from build123d import *

# Parameters (mm, degrees)
SKETCH1_W               = 300
SKETCH1_H               = 300
BOSS_EXTRUDE1_DEPTH     = 3
SKETCH2_W               = 300
SKETCH2_H               = 300
SKETCH2_W_2             = 294
SKETCH2_H_2             = 294
BOSS_EXTRUDE2_DEPTH     = 297
SKETCH3_W               = 300
SKETCH3_H               = 300
BOSS_EXTRUDE3_DEPTH     = 3
SKETCH4_R               = 25
CUT_EXTRUDE1_DEPTH      = 1
CUT_EXTRUDE1_DEPTH_BACK = 301
SKETCH5_W               = 300
SKETCH5_H               = 300
CUT_EXTRUDE2_DEPTH      = 3


with BuildPart() as part:
    # Sketch1 → Boss-Extrude1 (new body)
    with BuildSketch(Plane(origin=(0, 0, 0), x_dir=(1, 0, 0), z_dir=(0, 1, 0))):
        Rectangle(SKETCH1_W, SKETCH1_H)
    extrude(amount=BOSS_EXTRUDE1_DEPTH)

    # Sketch2 → Boss-Extrude2 (add)
    with BuildSketch(Plane(origin=(0, 3, 0), x_dir=(1, 0, 0), z_dir=(0, 1, 0))):
        Rectangle(SKETCH2_W, SKETCH2_H)
        Rectangle(SKETCH2_W_2, SKETCH2_H_2, mode=Mode.SUBTRACT)
    extrude(amount=BOSS_EXTRUDE2_DEPTH)

    # Sketch3 → Boss-Extrude3 (add)
    with BuildSketch(Plane(origin=(0, 300, 0), x_dir=(1, 0, 0), z_dir=(0, 1, 0))):
        Rectangle(SKETCH3_W, SKETCH3_H)
    extrude(amount=-BOSS_EXTRUDE3_DEPTH)

    # Sketch4 → Cut-Extrude1 (cut, two sides)
    with BuildSketch(Plane(origin=(150, 0, 0), x_dir=(0, 0, -1), z_dir=(1, 0, 0))) as cut_extrude1_sk:
        with Locations((0, 50)):
            Circle(SKETCH4_R)
    extrude(amount=CUT_EXTRUDE1_DEPTH, mode=Mode.SUBTRACT)
    extrude(cut_extrude1_sk.sketch, amount=-CUT_EXTRUDE1_DEPTH_BACK, mode=Mode.SUBTRACT)

    # Sketch5 → Cut-Extrude2 (cut)
    with BuildSketch(Plane.XZ):
        Rectangle(SKETCH5_W, SKETCH5_H)
    extrude(amount=-CUT_EXTRUDE2_DEPTH, mode=Mode.SUBTRACT)


solid = part.part
Design review of the part built by this model. Coordinates are the model's own, in mm. A direction names the side the tool comes from. Round coordinates to 2 decimals unless told otherwise and drop trailing zeros. Write each loop counter-clockwise with the first axis right and the second up, starting at its lowest first coordinate (ties: lowest second). Pieces come first, ordered by that corner, then holes. Notation, with made-up numbers: (85, 86) - (99, 86) arc R25 cw to (99, 113) - close; hole circle Ø5 at (-15.5, 79.25). An arc over 180 degrees is marked (long way). Return JSON: item names as keys, results as strings. Group by question number.
Item 1: We need section B-B on y = 50. Write out the cut boundary in (x, z), and give its area (3 significant figures).
Item 2: We need section D-D on y = 233. Write out the cut boundary in (x, z).
Item 3: The part is to be moulded in two halves that separate along Z. For faces 1 (the face through (-147, 148, 2)), 2 (the face through (-2, 149, 150)), 3 (the face through (-150, 149, 2)), say which applies: pulls with the +Z half, pulls with the -Z half, needs draft (parallel to the pull), parting line crosses it, or undercut.
Item 4: For probe 1 along X at (y, z) = (247, 42); probe 2 along Y at (x, z) = (-148, 0), list the stretches that pass through material, from the lowest coordinate up. Write a range as [from, to].
Item 5: We need section C-C on x = 23. Write out the cut boundary in (y, z), and give its area (3 significant figures).
Item 6: Insertion check: P1, Ø1, axis at x = 109.5, z = 83, coming from the -Y side. The pin has a flat end and moves straight along its axis. Give the tip position at first contact, or say it passes through.
Item 7: We need section A-A on z = 0. Write out the cut boundary in (x, y).
Item 8: Machinability: for faces 4 (the face through (150, 149, 2)), 5 (the face through (-2, 297, -2)), which of the approach directions +Z, -Z, +X, -X, +Y, -Y give a long, thin tool a straight path to every point of the face, cutting with its end or side? Answer none if there is none.
Model answer:
{
 "1": {"outline": "(-150, -150) - (150, -150) - (150, -25) - (147, -25) - (147, -147) - (-147, -147) - (-147, -25) - (-150, -25) - close; (-150, 25) - (-147, 25) - (-147, 147) - (147, 147) - (147, 25) - (150, 25) - (150, 150) - (-150, 150) - close", "area": "3,260 mm²"},
 "2": {"outline": "(-150, -150) - (150, -150) - (150, 150) - (-150, 150) - close; hole (-147, -147) - (147, -147) - (147, 147) - (-147, 147) - close"},
 "3": {"face 1": "undercut", "face 2": "pulls with the +Z half", "face 3": "needs draft"},
 "4": {"probe 1": "x = [-150, -147], [147, 150]", "probe 2": "y = [3, 25], [75, 300]"},
 "5": {"outline": "(3, -150) - (300, -150) - (300, 150) - (3, 150) - (3, 147) - (297, 147) - (297, -147) - (3, -147) - close", "area": "2,660 mm²"},
 "6": {"P1": "stops at y = 297"},
 "7": {"outline": "(-150, 3) - (-147, 3) - (-147, 25) - (-150, 25) - close; (-150, 75) - (-147, 75) - (-147, 297) - (147, 297) - (147, 75) - (150, 75) - (150, 300) - (-150, 300) - close; (147, 3) - (150, 3) - (150, 25) - (147, 25) - close"},
 "8": {"face 4": "+Z, -Z, +X, +Y, -Y", "face 5": "-Y"}
}
